Geometry: see drawing. Coordinates: mm, zero at the bounding-box minimum. Coordinates: 2 decimals unless noted, no trailing zeros. Order: outer loops, then holes, each group sorted by start corner. A loop starts at its lowest first (then second) coordinate and runs counter-clockwise, first axis right, second up. Notation, with made-up numbers: (-29, 66) - (1, 66) arc R30 ccw to (1, 90) - close; hole circle Ø10 at (20.25, 1). An arc over 180 degrees is marked (long way). Use a Markdown table: item, result. Add a question column.
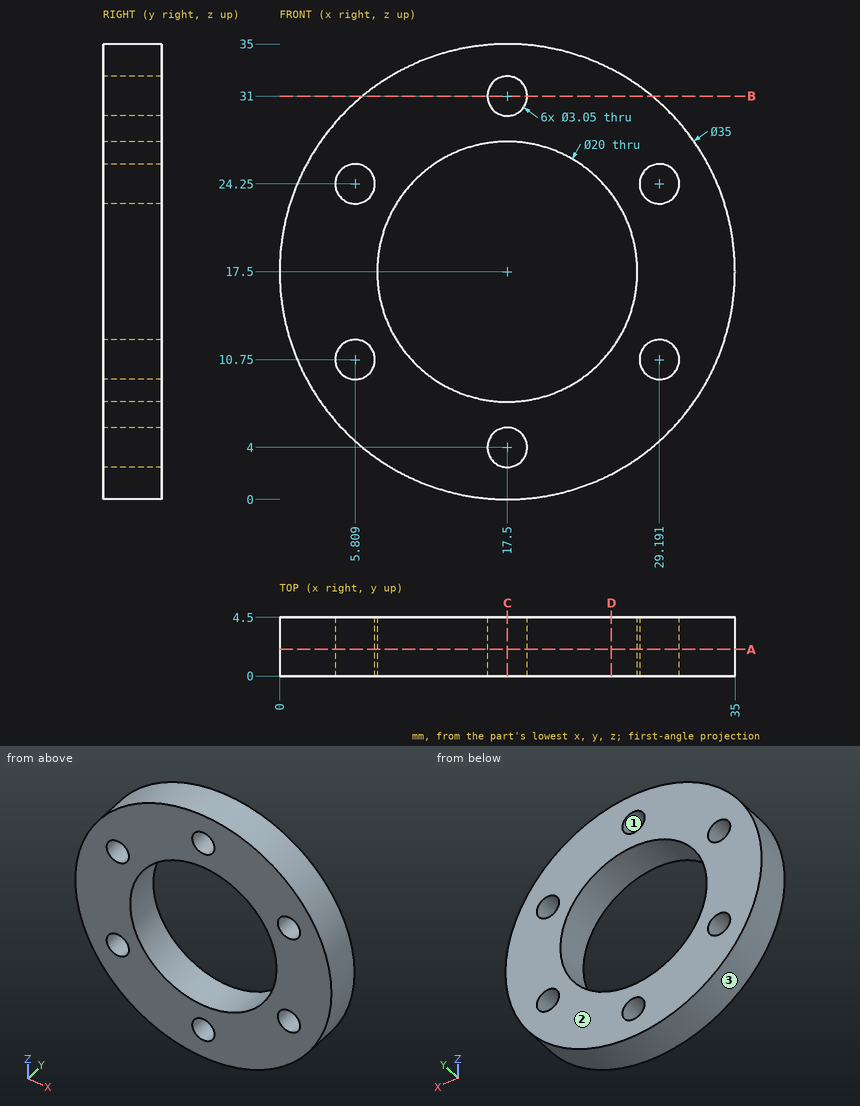
1) Cut plane D-D (x = 25.5). Return the cut outline in (y, z) (1 decimal).
2) Cut plane B-B (z = 31). Return the cut outline in (x, y) (1 decimal), and give its area (3 significant figures).
3) Cut plane A-A (y = 2.05). State how many separate pieces and enclosed holes the cut face has, and give its area (3 significant figures).
4) Cut plane C-C (x = 17.5). Return the cut outline in (y, z) (1 decimal).
5) Material intervals for L1, parallel to Z at x = 17.5, y = 3.05 (1 decimal); L2, parallel to X at y = 0.2, z = 24 (1 decimal); L3, parallel to Z at x = 4.5, y = 4.05 (1 decimal), sorted ascending.
6) Contact query for flat-ended pins moving along their axis: P1, Ø2, axis at y = 3.5, z = 13, coming from the +X side; P2, Ø1.5, axis at x = 5, y = 2.5, coming from the -Z side; P3, Ø1.8, axis at x = 29.19, z = 24.25, coming from the +Y side. Output: stop coordinate, or through.
7) Pull-direction query (Z, two-part tool) for the marked faces 1, 2 and 3; classes: pulls with the +Z half, pulls with the -Z half, needs draft (parallel to the pull), parting line crosses it, or undercut.
Computed:
| question | item | result |
|---|---|---|
| 1 | outline | (0, 1.9) - (4.5, 1.9) - (4.5, 11.5) - (0, 11.5) - close; (0, 23.5) - (4.5, 23.5) - (4.5, 33.1) - (0, 33.1) - close |
| 2 | outline | (6.4, 0) - (16, 0) - (16, 4.5) - (6.4, 4.5) - close; (19, 0) - (28.6, 0) - (28.6, 4.5) - (19, 4.5) - close |
| 2 | area | 86.5 mm2 |
| 3 | separate pieces | 1 |
| 3 | enclosed holes | 7 |
| 3 | area | 604 mm2 |
| 4 | outline | (0, 0) - (4.5, 0) - (4.5, 2.5) - (0, 2.5) - close; (0, 5.5) - (4.5, 5.5) - (4.5, 7.5) - (0, 7.5) - close; (0, 27.5) - (4.5, 27.5) - (4.5, 29.5) - (0, 29.5) - close; (0, 32.5) - (4.5, 32.5) - (4.5, 35) - (0, 35) - close |
| 5 | L1 | z = 0 to 2.5, 5.5 to 7.5, 27.5 to 29.5, 32.5 to 35 |
| 5 | L2 | x = 1.3 to 4.3, 7.3 to 9.9, 25.1 to 27.7, 30.7 to 33.7 |
| 5 | L3 | z = 5.8 to 10, 11.5 to 23.5, 25 to 29.2 |
| 6 | P1 | stops at x = 34.65 |
| 6 | P2 | stops at z = 4.53 |
| 6 | P3 | passes through |
| 7 | face 1 | undercut |
| 7 | face 2 | needs draft |
| 7 | face 3 | parting line crosses it |
